Geometry check sheet. Reference: the model listing, model coordinates, mm. A direction names the side the tool comes from. Give positions to 0.01 mm unless a question says otherwise; leave off trailing zeros. Write each loop counter-clockwise with the first axis right and the second up, starting at its lowest first coordinate (ties: lowest second). Pieces come first, ordered by that corner, then holes. Notation, with made-up numbers: (29, 49.25) - (50, 49.25) arc R35 cw to (50, 85.25) - close; hole circle Ø9 at (22.5, 29). An arc over 180 degrees is marked (long way). Use a Markdown table: item, result.
```python
from build123d import *

# Parameters (mm, degrees)
F0_R           = 4.58966
F1_DEPTH       = 9.525
F2_R           = 4.58966
F3_DEPTH       = 6.35
F5_D           = 4.7625
F5_DEPTH       = 12.7
F5_CBORE_D     = 6.35
F5_CBORE_DEPTH = 3.175


with BuildPart() as f1:
    # F0 (on Top) → F1 (new body)
    with BuildSketch(Plane.XY):
        with BuildLine():
            Line((31.311959, 7.866156), (36.626371, 11.336331))
            ThreePointArc((36.626371, 11.336331), (39.257746, 23.870263), (26.723814, 26.501637))
            Line((26.723814, 26.501637), (16.431446, 19.780984))
            ThreePointArc((16.431446, 19.780984), (16.032886, 19.596337), (15.598217, 19.533035))
            Line((15.598217, 19.533035), (2.571234, 19.533035))
            ThreePointArc((2.571234, 19.533035), (-16.700992, 1.336157), (-35.973218, 19.533035))
            Line((-35.973218, 19.533035), (-51.14509, 19.533035))
            ThreePointArc((-51.14509, 19.533035), (-52.22272, 19.086666), (-52.66909, 18.009035))
            Line((-52.66909, 18.009035), (-52.66909, 8.357035))
            ThreePointArc((-52.66909, 8.357035), (-52.22272, 7.279404), (-51.14509, 6.833035))
            Line((-51.14509, 6.833035), (-41.62009, 6.833035))
            ThreePointArc((-41.62009, 6.833035), (-39.04111, 6.285738), (-36.906687, 4.738189))
            Line((-36.906687, 4.738189), (-29.993949, -2.918997))
            ThreePointArc((-29.993949, -2.918997), (-27.859527, -4.466546), (-25.280547, -5.013843))
            Line((-25.280547, -5.013843), (-8.121436, -5.013843))
            ThreePointArc((-8.121436, -5.013843), (-5.542457, -4.466546), (-3.408034, -2.918997))
            Line((-3.408034, -2.918997), (4.942001, 6.330272))
            ThreePointArc((4.942001, 6.330272), (5.454262, 6.701684), (6.073217, 6.833035))
            Line((6.073217, 6.833035), (27.840173, 6.833035))
            ThreePointArc((27.840173, 6.833035), (29.651294, 7.096793), (31.311959, 7.866156))
        make_face()
        with Locations((31.675093, 18.918984)):
            Circle(F0_R, mode=Mode.SUBTRACT)
    extrude(amount=F1_DEPTH)

    # F2 (on face) → F3 (cut)
    with BuildSketch(Plane(origin=(0, 0, 0), x_dir=(1, 0, 0), z_dir=(0, 0, -1))):
        with BuildLine():
            Line((27.840173, -6.833035), (16.431446, -19.780984))
            Line((16.431446, -19.780984), (26.723814, -26.501637))
            ThreePointArc((26.723814, -26.501637), (39.257746, -23.870263), (36.626371, -11.336331))
            Line((36.626371, -11.336331), (31.311959, -7.866156))
            ThreePointArc((31.311959, -7.866156), (29.651294, -7.096793), (27.840173, -6.833035))
        make_face()
        with Locations((31.675093, -18.918984)):
            Circle(F2_R, mode=Mode.SUBTRACT)
    extrude(amount=-F3_DEPTH, mode=Mode.SUBTRACT)

    # F5
    with Locations(Plane.XZ.offset(-6.833035)):
        with Locations((-46.38259, 4.7625), (10.835717, 4.74801)):
            CounterBoreHole(F5_D / 2, F5_CBORE_D / 2, F5_CBORE_DEPTH, depth=F5_DEPTH)


solid = f1.part
```
1) Set-up check for faces 1 (the cylindrical face through (8.5, 8.4, 6.9)), 2 (the flat face through (22.216, 13.216, 3.131)), 3 (the flat face through (-50, 6.833, 5)), 4 (the flat face through (8, 19.533, 5)): record each of +Z, -Z, +X, -X, +Y, -Y from which the full face is reachable in a straight line by a thin tool's end or side.
Working result:
| item | result |
|---|---|
| face 1 | -Y |
| face 2 | -Z, +X, +Y |
| face 3 | +Z, -Z, -X, -Y |
| face 4 | +Z, -Z, -X, +Y |
2) Mould release check, pull along Z, two halves, no side actions. Record for faces 5 (the flat face through (12, 10.008, 7)), 6 (the flat face through (33.932, 9.577, 7.915)), 7 (the flat face through (28, 15, 6.35)): pulls with the +Z half, pulls with the -Z half, needs draft (parallel to the pull), parting line crosses it, or undercut.
Working result:
| item | result |
|---|---|
| face 5 | undercut |
| face 6 | needs draft |
| face 7 | pulls with the -Z half |
3) Section check A-A on y = 3. Record the boundary of the cut face in (x, z) (1 decimal).
Working result:
| item | result |
|---|---|
| outline | (-35.3, 0) - (-24.5, 0) - (-24.5, 9.5) - (-35.3, 9.5) - close; (-8.9, 0) - (1.9, 0) - (1.9, 9.5) - (-8.9, 9.5) - close |
4) Section check C-C on x = 32.5. Record the boundary of the cut face in (y, z) (3 decimals).
Working result:
| item | result |
|---|---|
| outline | (8.642, 6.35) - (14.404, 6.35) - (14.404, 9.525) - (8.642, 9.525) - close; (23.434, 6.35) - (27.937, 6.35) - (27.937, 9.525) - (23.434, 9.525) - close |
5) Section check D-D on x = -14. Record the boundary of the cut face in (y, z) (3 decimals).
Working result:
| item | result |
|---|---|
| outline | (-5.014, 0) - (1.526, 0) - (1.526, 9.525) - (-5.014, 9.525) - close |
6) Section check B-B on z = 3.25. Count the separate pieces of the cut face and the enclosed holes in it, then the cut area to 3 significant figures.
Working result:
| item | result |
|---|---|
| separate pieces | 3 |
| enclosed holes | 0 |
| area | 698 mm² |
7) Material ranges on L1, parallel to X at y = 7.5, z = 2; L2, parallel to X at y = 9.5, z = 6.5; L3, parallel to Y at x = 15.5, z = 7.75, recorded low to high. Write a range as from..to.
Working result:
| item | result |
|---|---|
| L1 | x = -52.41..-47.95, -44.82..-30.84, -2.56..9.25, 12.43..27.25 |
| L2 | x = -52.67..-49.04, -43.73..-32.47, -0.94..8.19, 13.48..33.81 |
| L3 | y = 6.83..19.53 |
8) Depth check by flat-ended pin: P1, Ø5, axis at x = 10.84, z = 4.75, coming from the +Y side; P2, Ø3, axis at x = 29, z = 7, coming from the +Y side; P3, Ø3, axis at x = 10.5, z = 3.5, coming from the -Y side. Enter the tip coordinate at first touch or a pass-through.
Working result:
| item | result |
|---|---|
| P1 | stops at y = 19.53 |
| P2 | stops at y = 27.9 |
| P3 | stops at y = 10.01 |
